The listing builds one solid part. Answer for the finished solid, in the listing's coordinates (mm). Round coordinates to 2 decimals unless told otherwise and drop trailing zeros. Order: outer loops, then holes, each group sorted by start corner. A loop starts at its lowest first (then second) coordinate and runs counter-clockwise, first axis right, second up. Notation, with made-up numbers: M 28,21 L 83,21 A26 ccw 83,45 Z; hole C 6.25,-34 d4. An arc over 180 degrees is marked long. Put each result on its own line as item: value. Start each with the question number.
1. The part is cut by section A-A (z = 6.5). Give the vertices of the cut face in (x, y).
2. This flat-tipped pin is pushed along its axis until it touches: pin 1 Ø6 at (y, z) = (-257, 1) entering from +X. Where does it stop, or does it pass through?
3. The part is cut by section B-B (y = -346). Give the vertices of the cut face in (x, z).
4. Consider line 1 (Y direction, x = 0, z = 7.5); line 2 (X direction, y = -387, z = 4); line 3 (Y direction, x = -2.5, z = 4.5). Determine where each line is inside the solid, lowest interval first.
5. The part is cut by section C-C (x = 23). Give the vertices of the cut face in (y, z).
from build123d import *

# Parameters (mm, degrees)
SKETCH1_R           = 3
BOSS_EXTRUDE1_DEPTH = 10
SKETCH2_R           = 3
BOSS_EXTRUDE3_DEPTH = 10


with BuildPart() as part:
    # Sketch1 → Boss-Extrude1 (new body)
    with BuildSketch(Plane.XY):
        with BuildLine():
            Line((-12.5, 0), (-12.5, -500))
            ThreePointArc((-12.5, -500), (0, -512.5), (12.5, -500))
            Line((12.5, -500), (12.5, 0))
            ThreePointArc((12.5, 0), (0, 12.5), (-12.5, 0))
        make_face()
        Circle(SKETCH1_R, mode=Mode.SUBTRACT)
        with Locations(Location((0, -500, 0), (0, 0, 180))):
            Circle(SKETCH1_R, mode=Mode.SUBTRACT)
    extrude(amount=BOSS_EXTRUDE1_DEPTH)

    # Sketch2 → Boss-Extrude3 (add)
    with BuildSketch(Plane.XY.offset(10)):
        Polygon((12.5, -488.503824236), (78.810550707, -567.529661268), (59.659439629, -583.59935151), (0, -512.5), align=None)
        with Locations((61.200150047, -565.98895085)):
            Circle(SKETCH2_R, mode=Mode.SUBTRACT)
    extrude(amount=-BOSS_EXTRUDE3_DEPTH)


solid = part.part
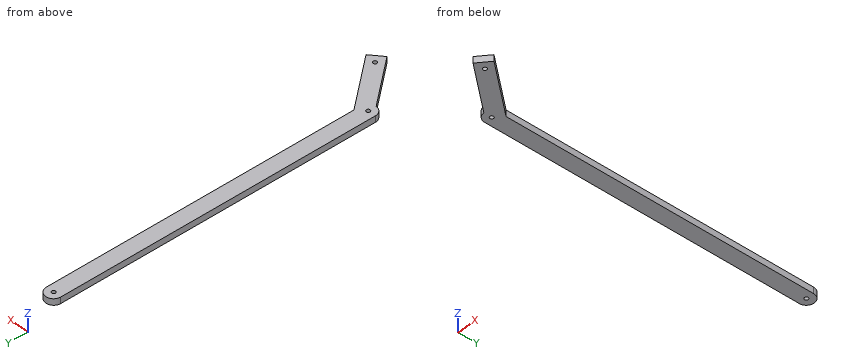
Resolved:
1. outline: M -12.5,-500 A12.5 ccw 0,-512.5 L 59.66,-583.6 L 78.81,-567.53 L 12.5,-488.5 L 12.5,0 A12.5 ccw -12.5,0 Z; hole C 0,-500 d6; hole C 0,0 d6; hole C 61.2,-565.99 d6
2. pin 1: x = 12.5
3. outline: M -12.5,0 L 12.5,0 L 12.5,10 L -12.5,10 Z
4. line 1: -512.5 to -503, -497 to -3, 3 to 12.5
4. line 2: -12.5 to 12.5
4. line 3: -512.25 to -501.66, -498.34 to -1.66, 1.66 to 12.25
5. outline: M -539.91,0 L -501.02,0 L -501.02,10 L -539.91,10 Z
